Check sheet for the modelled part. Datum: model origin and axes. Units: mm. A direction names the side the tool comes from. Give positions to 0.01 mm unless a question says otherwise; leave off trailing zeros. Order: outer loops, then holes, each group sorted by start corner. A loop starts at its lowest first (then second) coordinate and runs counter-clockwise, first axis right, second up.
Item 1: Sectioned sample at B-B on x = 0. Record the boundary of the cut face in (y, z).
Item 2: Sectioned sample at A-A on z = 0. Record the boundary of the cut face in (x, y).
Item 3: Material ranges on line 1 along X through (y, z) = (19, 0); line 2 along Y through (x, z) = (11, -2); line 3 along X through (y, z) = (22, -8.5), recorded low to high.
Item 4: Access from +Z, -Z, +X, -X, +Y, -Y to the whole of each face (thin tool, end or side, straight path). Record for faces 4 (the cylindrical face through (-0.6, 15.6, -9.3)), 5 (the cylindrical face through (-3.417, 31.934, -0.759)).
Item 5: Sectioned sample at C-C on y = 9. Record the boundary of the cut face in (x, z), and give its area (3 significant figures).
Item 6: Release check for a two-part mould opening along Z. For faces 1 (the cylindrical face through (4.654, 15.691, -11.224)), 2 (the flat face through (0, 0, 2)), 3 (the cylindrical face through (-1.71, 16.78, -0.38)) record: released by +Z, released by -Z, zero draft, split by the parting line, or undercut.
Item 7: Gauge pin test, flat ends, axial feed: P1, Ø3, axis at y = 13.5, z = -7, coming from the -X side; P2, Ø6, axis at x = 4, z = 0, coming from the +Y side; P3, Ø1.5, axis at y = 15.5, z = -9.5, coming from the -X side; P4, Ø1.5, axis at y = 12, z = 1.5, coming from the +X side. Record the tip position at first contact, or that the pin passes through.
from build123d import *

# Parameters (mm, degrees)
SKETCH_1_R           = 12.15
EXTRUDE_1_DEPTH      = 30.8
FILLET_1_R           = 1
EXTRUDE_2_DEPTH      = 2.3
EXTRUDE_2_DEPTH_BACK = 30.8
SKETCH_2_R           = 3.5
SKETCH_3_R           = 1
CUT_EXTRUDE_1_DEPTH  = 36.268753911
SKETCH_4_R           = 1.75
CUT_EXTRUDE_2_DEPTH  = 38.294168478


with BuildPart() as part:
    # 草图1 → 凸台-拉伸1 (new body)
    with BuildSketch(Plane(origin=(0, 0, 0), x_dir=(1, 0, 0), z_dir=(0, 1, 0))):
        with Locations(Location((0, 0, 0), (0, 0, 90))):
            Circle(SKETCH_1_R)
    extrude(amount=EXTRUDE_1_DEPTH)

    # 圆角1
    fillet_1_edges = [part.edges().sort_by_distance(p)[0] for p in [
        (0, 0, 12.15),
    ]]
    fillet(fillet_1_edges, radius=FILLET_1_R)

    # 草图2 → 凸台-拉伸2 (add, two sides: drawn at the far end of the back side and taken through both)
    with BuildSketch(Plane(origin=(0, 30.8, 0), x_dir=(1, 0, 0), z_dir=(0, 1, 0)).offset(-EXTRUDE_2_DEPTH_BACK)):
        with Locations(Location((0, 0, 0), (0, 0, 270))):
            Circle(SKETCH_2_R)
    extrude(amount=EXTRUDE_2_DEPTH + EXTRUDE_2_DEPTH_BACK)

    # 草图3 → 切除-拉伸1 (cut, through all)
    with BuildSketch(Plane(origin=(0, 30.8, 0), x_dir=(1, 0, 0), z_dir=(0, 1, 0))):
        with Locations(Location((0, 8.5, 0), (0, 0, 270))):
            Circle(SKETCH_3_R)
        with Locations(Location((0, -8.5, 0), (0, 0, 270))):
            Circle(SKETCH_3_R)
    extrude(amount=-CUT_EXTRUDE_1_DEPTH, mode=Mode.SUBTRACT)

    # 草图4 → 切除-拉伸2 (cut, through all)
    with BuildSketch(Plane(origin=(0, 33.1, 0), x_dir=(1, 0, 0), z_dir=(0, 1, 0))):
        with Locations(Location((0, 0, 0), (0, 0, 270))):
            Circle(SKETCH_4_R)
    extrude(amount=-CUT_EXTRUDE_2_DEPTH, mode=Mode.SUBTRACT)


solid = part.part
Report:
1. outline: (0, -11.15) arc R1 ccw to (1, -12.15) - (30.8, -12.15) - (30.8, -9.5) - (0, -9.5) - close; (0, -7.5) - (30.8, -7.5) - (30.8, -3.5) - (33.1, -3.5) - (33.1, -1.75) - (0, -1.75) - close; (0, 1.75) - (33.1, 1.75) - (33.1, 3.5) - (30.8, 3.5) - (30.8, 7.5) - (0, 7.5) - close; (0, 9.5) - (30.8, 9.5) - (30.8, 12.15) - (1, 12.15) arc R1 ccw to (0, 11.15) - close
2. outline: (-12.15, 1) arc R1 ccw to (-11.15, 0) - (-1.75, 0) - (-1.75, 33.1) - (-3.5, 33.1) - (-3.5, 30.8) - (-12.15, 30.8) - close; (1.75, 0) - (11.15, 0) arc R1 ccw to (12.15, 1) - (12.15, 30.8) - (3.5, 30.8) - (3.5, 33.1) - (1.75, 33.1) - close
3. line 1: x = -12.15 to -1.75, 1.75 to 12.15
3. line 2: y = 0 to 30.8
3. line 3: x = -8.68 to -1, 1 to 8.68
4. face 4: +Y, -Y
4. face 5: +Y
5. outline: circle Ø24.3 at (0, 0); hole circle Ø3.5 at (0, 0); hole circle Ø2 at (0, -8.5); hole circle Ø2 at (0, 8.5)
5. area: 448 mm2
6. face 1: split by the parting line
6. face 2: zero draft
6. face 3: undercut
7. P1: stops at x = -10.83
7. P2: stops at y = 33.1
7. P3: stops at x = -8.43
7. P4: stops at x = 12.13
